Geometry check sheet. Reference: drawing and pictorial views, mm from the part's lowest x, y, z. A direction names the side the tool comes from. Round coordinates to 2 decimals unless told otherwise and drop trailing zeros. Write each loop counter-clockwise with the first axis right and the second up, starting at its lowest first coordinate (ties: lowest second). Pieces come first, ordered by that corner, then holes. Notation, with made-up numbers: (-36.5, -11.75) - (-29.5, -11.75) arc R18 cw to (-29.5, 5.25) - close; hole circle Ø7 at (-9.75, -6.75). An arc over 180 degrees is marked (long way). Use one line per item in the form item = value. Start each with the question number.
1) Section check C-C (z = 4.25). Record the boundary of the cut face in (x, y).
2) Draft check along Z on the marked faces 4, 5 and 6. Enter one of: +Z half, -Z half, draft (parallel to the pull), parting line (faces both ways), or undercut.
3) Set-up check for the marked faces 1, 2 and 3: record each of +Z, -Z, +X, -X, +Y, -Y from which the full face is reachable in a straight line by a thin tool's end or side.
4) Section check D-D (x = 10.5). Record the boundary of the cut face in (y, z).
5) Gauge pin test, flat ends, axial feed: P1, Ø0.6, axis at y = 1, z = 3.5, coming from the -X side; P2, Ø1.9, axis at x = 10, y = 6, coming from the -Z side; P3, Ø1.5, axis at y = 3, z = 1, coming from the +X side; P4, Ø4, axis at x = 11, z = 6.5, coming from the +Y side. Record the tip position at first contact, or that the pin passes through.
6) Scan lines: probe 1 along X at (y, z) = (1.5, 3.75); probe 2 along X at (y, z) = (0.5, 7.75); probe 3 along Z at (x, y) = (2.25, 0.5). Record each from-to range of solid material in increasing order.
7) Section check B-B (y = 4.25). Record the boundary of the cut face in (x, z).
8) Section check A-A (x = 17). Record the boundary of the cut face in (y, z).
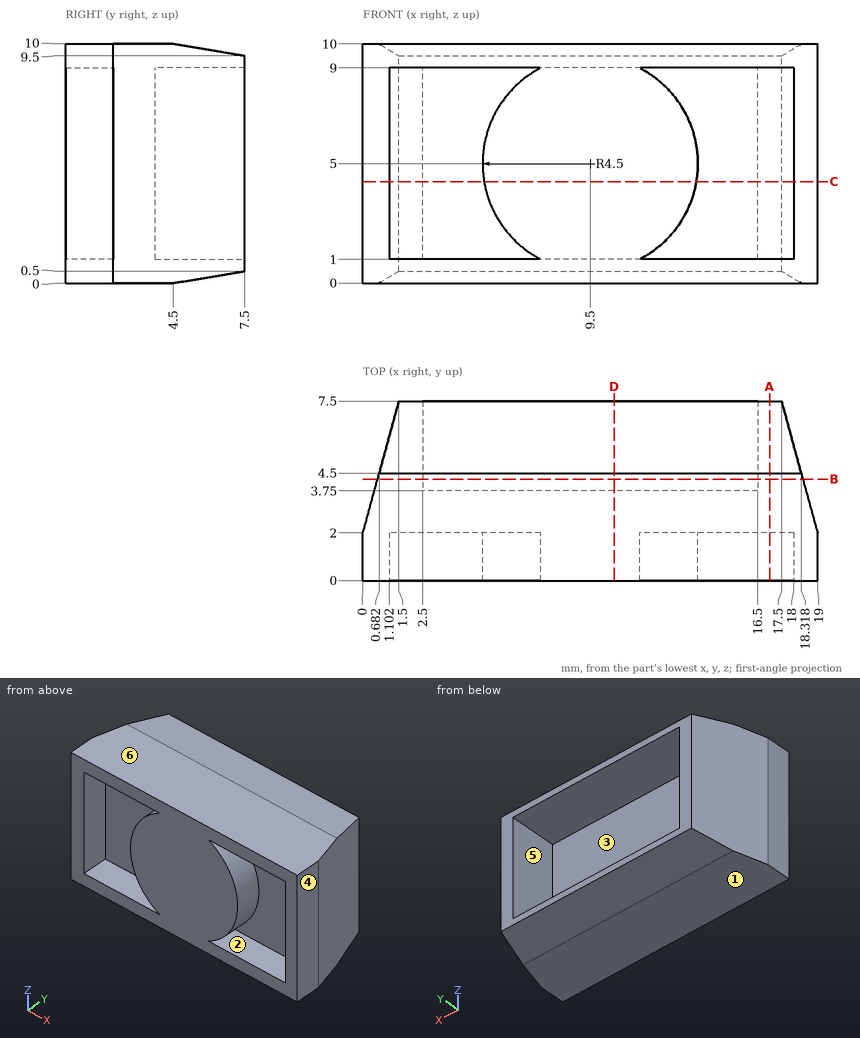
Results are:
q1.outline = (0, 0) - (1.1, 0) - (1.1, 2) - (5.06, 2) - (5.06, 0) - (13.94, 0) - (13.94, 2) - (18, 2) - (18, 0) - (19, 0) - (19, 2) - (17.5, 7.5) - (16.5, 7.5) - (16.5, 3.75) - (2.5, 3.75) - (2.5, 7.5) - (1.5, 7.5) - (0, 2) - close
q2.face_4 = draft
q2.face_5 = undercut
q2.face_6 = +Z half
q3.face_1 = -Z, +X, -X, +Y, -Y
q3.face_2 = -Y
q3.face_3 = +Y
q4.outline = (0, 0) - (4.5, 0) - (7.5, 0.5) - (7.5, 1) - (3.75, 1) - (3.75, 9) - (7.5, 9) - (7.5, 9.5) - (4.5, 10) - (0, 10) - close
q5.P1 = 0
q5.P2 = 0.09
q5.P3 = 18.93
q5.P4 = 3.75
q6.probe_1 = 0 to 1.1, 5.18 to 13.82, 18 to 19
q6.probe_2 = 0 to 1.1, 5.94 to 13.06, 18 to 19
q6.probe_3 = 0 to 1, 9 to 10
q7.outline = (0.61, 0) - (18.39, 0) - (18.39, 10) - (0.61, 10) - close; hole (2.5, 1) - (16.5, 1) - (16.5, 9) - (2.5, 9) - close
q8.outline = (0, 0) - (4.5, 0) - (7.5, 0.5) - (7.5, 9.5) - (4.5, 10) - (0, 10) - (0, 9) - (2, 9) - (2, 1) - (0, 1) - close
